```python
from build123d import *

# Parameters (mm, degrees)
SKETCH1_W           = 121.11
SKETCH1_H           = 77.93
SKETCH1_R           = 1.454399876
BOSS_EXTRUDE1_DEPTH = 1.5875
SKETCH2_W           = 120.91
SKETCH2_H           = 76.529195788
BOSS_EXTRUDE2_DEPTH = 3
SKETCH3_W           = 116.91
SKETCH3_H           = 72.029195788
BOSS_EXTRUDE3_DEPTH = 1


with BuildPart() as part:
    # Sketch1 → Boss-Extrude1 (new body)
    # profile 1 of 5: a face of its own
    with BuildSketch(Plane.XY):
        Rectangle(SKETCH1_W, SKETCH1_H)
    # profile 2 of 5: a face of its own
    with BuildSketch(Plane.XY):
        with BuildLine():
            Line((54.535, 42.225), (54.535, 38.965))
            Line((54.535, 38.965), (60.555, 38.965))
            Line((60.555, 38.965), (60.555, 42.225))
            ThreePointArc((60.555, 42.225), (59.822766953, 43.992766953), (58.055, 44.725))
            Line((58.055, 44.725), (57.035, 44.725))
            ThreePointArc((57.035, 44.725), (55.267233047, 43.992766953), (54.535, 42.225))
        make_face()
        with Locations((57.545, 41.845)):
            Circle(SKETCH1_R, mode=Mode.SUBTRACT)
    # profile 3 of 5: a face of its own
    with BuildSketch(Plane.XY):
        with BuildLine():
            Line((60.555, -38.965), (54.535, -38.965))
            Line((54.535, -38.965), (54.535, -42.225))
            ThreePointArc((54.535, -42.225), (55.267233047, -43.992766953), (57.035, -44.725))
            Line((57.035, -44.725), (58.055, -44.725))
            ThreePointArc((58.055, -44.725), (59.822766953, -43.992766953), (60.555, -42.225))
            Line((60.555, -42.225), (60.555, -38.965))
        make_face()
        with Locations((57.545, -41.845)):
            Circle(SKETCH1_R, mode=Mode.SUBTRACT)
    # profile 4 of 5: a face of its own
    with BuildSketch(Plane.XY):
        with BuildLine():
            Line((-60.555, 42.225), (-60.555, 38.965))
            Line((-60.555, 38.965), (-54.535, 38.965))
            Line((-54.535, 38.965), (-54.535, 42.225))
            ThreePointArc((-54.535, 42.225), (-55.267233047, 43.992766953), (-57.035, 44.725))
            Line((-57.035, 44.725), (-58.055, 44.725))
            ThreePointArc((-58.055, 44.725), (-59.822766953, 43.992766953), (-60.555, 42.225))
        make_face()
        with Locations((-57.545, 41.845)):
            Circle(SKETCH1_R, mode=Mode.SUBTRACT)
    # profile 5 of 5: a face of its own
    with BuildSketch(Plane.XY):
        with BuildLine():
            Line((-54.535, -38.965), (-60.555, -38.965))
            Line((-60.555, -38.965), (-60.555, -42.225))
            ThreePointArc((-60.555, -42.225), (-59.822766953, -43.992766953), (-58.055, -44.725))
            Line((-58.055, -44.725), (-57.035, -44.725))
            ThreePointArc((-57.035, -44.725), (-55.267233047, -43.992766953), (-54.535, -42.225))
            Line((-54.535, -42.225), (-54.535, -38.965))
        make_face()
        with Locations((-57.545, -41.845)):
            Circle(SKETCH1_R, mode=Mode.SUBTRACT)
    extrude(amount=BOSS_EXTRUDE1_DEPTH)

    # Sketch2 → Boss-Extrude2 (add)
    with BuildSketch(Plane.XY.offset(1.5875)):
        with Locations((0, -0.600402106)):
            Rectangle(SKETCH2_W, SKETCH2_H)
    extrude(amount=BOSS_EXTRUDE2_DEPTH)

    # Sketch3 → Boss-Extrude3 (add)
    with BuildSketch(Plane.XY.offset(4.5875)):
        with Locations((0, 0.649597894)):
            Rectangle(SKETCH3_W, SKETCH3_H)
    extrude(amount=BOSS_EXTRUDE3_DEPTH)


solid = part.part
```
Source: CAD feature listing. Evaluate the final solid. Frame: model axes, mm. A direction names the side the tool comes from. Give positions to 0.01 mm unless a question says otherwise; leave off trailing zeros. Loops run counter-clockwise (first coordinate to the right, second up) from the corner with the lowest first, then second, coordinate; pieces in that order, holes last. Notation, with made-up numbers: (-30.75, 77.5) -> (10.25, 77.5) arc R20 ccw to (10.25, 97.5) -> close; hole circle Ø9 at (80.5, 2.25). An arc over 180 degrees is marked (long way). Use a Markdown table: item, result. Add a question column.
(1) Section query B-B (z = 3.6). Output: boundary loops of the cut face in (x, y) (3 decimals).
(2) Ray query, line 1 (Z direction, x = 18, y = 37); line 2 (Y direction, x = 31.5, z = 2.1) (3 decimals); line 3 (X direction, y = 16, z = 3.25) (3 decimals). Return the intervals inside material, ascending.
(3) First-contact query: pin 1 Ø0.8 at (x, z) = (-3.5, 0.5) entering from -Y (3 decimals); pin 2 Ø1.5 at (y, z) = (5, 3) entering from -X (3 decimals); pin 3 Ø0.9 at (x, z) = (-12, 4) entering from +Y. Flat tips, straight axial feed; report the tip coordinate or a pass-through.
(4) Pull-direction query (Y, two-part tool) for faces 1 (the face through (58.932, -41.408, 0.783)), 2 (the face through (-1, -38.865, 3)), 3 (the face through (-1, 1, 0)); classes: +Y half, -Y half, draft (parallel to the pull), parting line (faces both ways), or undercut.
(5) Access query for faces 4 (the face through (-60.455, -1, 3)), 5 (the face through (60.455, -1, 3)), 6 (the face through (-55.287, -44.012, 0.783)), 7 (the face through (-56.158, 42.282, 0.783)), 8 (the face through (-55.248, 43.973, 0.783)). Directions: +Z, -Z, +X, -X, +Y, -Y. A direction counts if a zero-diameter tool reaches every point of the face in a straight line with its end or side. Return the directions, or none.
Checked values:
| question | item | result |
|---|---|---|
| 1 | outline | (-60.455, -38.865) -> (60.455, -38.865) -> (60.455, 37.664) -> (-60.455, 37.664) -> close |
| 2 | line 1 | 0 to 4.59 |
| 2 | line 2 | -38.865 to 37.664 |
| 2 | line 3 | -60.455 to 60.455 |
| 3 | pin 1 | y = -38.965 |
| 3 | pin 2 | x = -60.455 |
| 3 | pin 3 | y = 37.66 |
| 4 | face 1 | undercut |
| 4 | face 2 | -Y half |
| 4 | face 3 | draft |
| 5 | face 4 | +Z, -X, +Y, -Y |
| 5 | face 5 | +Z, +X, +Y, -Y |
| 5 | face 6 | +Z, -Z, -Y |
| 5 | face 7 | +Z, -Z |
| 5 | face 8 | +Z, -Z, +Y |
